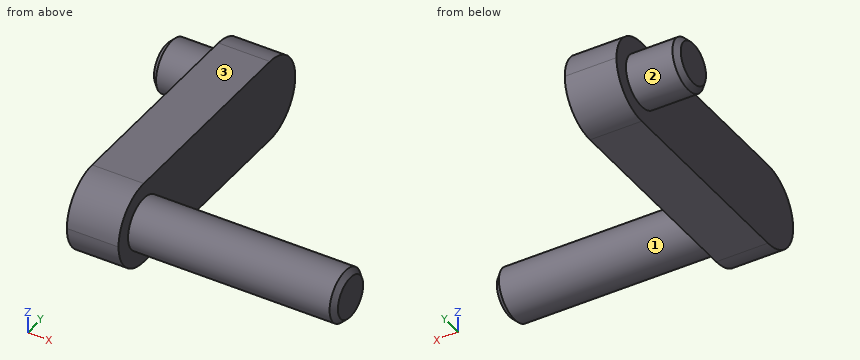
```python
from build123d import *

# Parameters (mm, degrees)
F0_R          = 2.5
F1_DEPTH      = 25
F2_DEPTH      = 5
F3_DEPTH      = 5
F3_DEPTH_BACK = 5
F4_SIZE       = 0.5


with BuildPart() as f1:
    # F0 (on Right) → F1 (new body)
    with BuildSketch(Plane.YZ):
        with Locations((4, 0)):
            Circle(F0_R)
    extrude(amount=F1_DEPTH)

    # F0 (on Right) → F2 (join)
    with BuildSketch(Plane.YZ):
        with BuildLine():
            ThreePointArc((0, 0), (1.1715728753, -2.8284271247), (4, -4))
            Line((4, -4), (24, -4))
            ThreePointArc((24, -4), (26.8284271247, -2.8284271247), (28, 0))
            ThreePointArc((28, 0), (26.8284271247, 2.8284271247), (24, 4))
            Line((24, 4), (4, 4))
            ThreePointArc((4, 4), (1.1715728753, 2.8284271247), (0, 0))
        make_face()
        with Locations((4, 0)):
            Circle(F0_R, mode=Mode.SUBTRACT)
        with Locations((24, 0)):
            Circle(F0_R, mode=Mode.SUBTRACT)
    extrude(amount=F2_DEPTH)

    # F0 (on Right) → F3 (join, two sides)
    with BuildSketch(Plane.YZ) as f3_sk:
        with Locations((24, 0)):
            Circle(F0_R)
    extrude(amount=-F3_DEPTH)
    extrude(f3_sk.sketch, amount=F3_DEPTH_BACK)

    # F4
    f4_edges = [f1.edges().sort_by_distance(p)[0] for p in [
        (-5, 21.5, 0),
        (25, 1.5, 0),
    ]]
    chamfer(f4_edges, length=F4_SIZE)


solid = f1.part
```
Input: part model. Units: mm. Frame: model coordinates. Face numbers are marked on the shaded views. A direction names the side the tool comes from. Coordinates: 2 decimals unless noted, no trailing zeros. Loops run counter-clockwise (first coordinate to the right, second up) from the corner with the lowest first, then second, coordinate; pieces in that order, holes last. Notation, with made-up numbers: M 47.25,70.25 L 86.25,70.25 A23 cw 86.25,88.25 Z; hole C 53.25,-21.75 d1. An arc over 180 degrees is marked long. One line per item, written item: value.
(1) Pin query (flat end, axial travel): pin 1 (1 mm diameter, centred on x = 11, z = -0.5, fed in from +Y); pin 2 (2 mm diameter, centred on y = 3.5, z = 2, fed in from -X); pin 3 (3 mm diameter, centred on y = 15.5, z = 2.5, fed in from +X); pin 4 (1.5 mm diameter, centred on x = 7.5, y = 17.5, fed in from +Z). Return the tip coordinate at first contact, or that it passes through.
Filled in:
pin 1: y = 6.5
pin 2: x = 0
pin 3: x = 5
pin 4: through
(2) Line query: line 1 along Y through (x, z) = (20.75, 1.5); line 2 along X through (y, z) = (12, -2.25); line 3 along X through (y, z) = (25.75, -0.5). Output: solid intervals per line, ascending. Write a range as from..to.
Filled in:
line 1: 2..6
line 2: 0..5
line 3: -5..5
(3) Reachability of the marked faces 1, 2 and 3 from +Z, -Z, +X, -X, +Y, -Y: full face, straight path, thin tool, end or side. Return the list, or none.
Filled in:
face 1: +X
face 2: -X
face 3: +Z, +X, -X, +Y, -Y
(4) Section A-A (x = 1.5). Output: boundary loops of the cut face in (y, z).
Filled in:
outline: M 4,-4 L 24,-4 A4 ccw 24,4 L 4,4 A4 ccw Z
(5) Section C-C (x = 20.5). Output: boundary loops of the cut face in (y, z).
Filled in:
outline: C 4,0 d5
(6) Section B-B (y = 7). Output: boundary loops of the cut face in (x, z).
Filled in:
outline: M 0,-4 L 5,-4 L 5,4 L 0,4 Z
